The model under review builds one solid part; all positions refer to its coordinate system, in mm. Face numbers are marked on the shaded views. A direction names the side the tool comes from. Coordinates: 2 decimals unless noted, no trailing zeros. Order: outer loops, then holes, each group sorted by start corner. A loop starts at its lowest first (then second) coordinate and runs counter-clockwise, first axis right, second up. Notation, with made-up numbers: M 14,72 L 61,72 A14 cw 61,93 Z; hole C 41,-14.75 d4. An arc over 180 degrees is marked long. One line per item, written item: value.
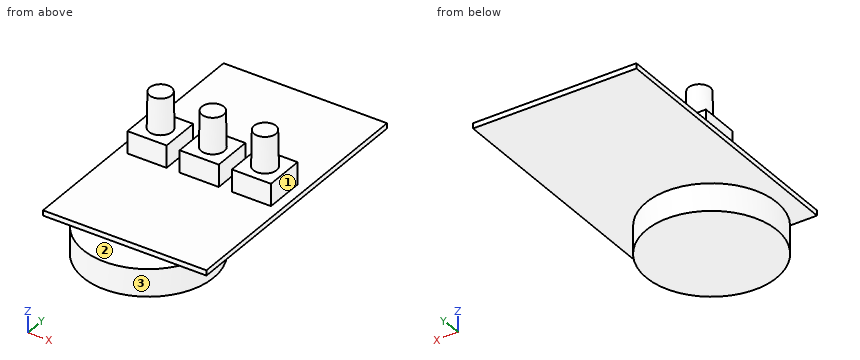
```python
from build123d import *

# Parameters (mm, degrees)
SKETCH_20_W                   = 25.05
SKETCH_20_H                   = 41.23
BOSS_EXTRUDE1_DEPTH           = 0.8
SKETCH13_W                    = 6
SKETCH13_H                    = 6.063806384
BOSS_EXTRUDE2_DEPTH           = 3.4
SKETCH14_R                    = 1.778
BOSS_EXTRUDE3_DEPTH           = 5.5
BOSS_EXTRUDE3_DRAFT           = 1
BOSS_EXTRUDE3_PROFILE_2_DEPTH = 5.5
BOSS_EXTRUDE3_PROFILE_2_DRAFT = 1
BOSS_EXTRUDE3_PROFILE_3_DEPTH = 5.5
BOSS_EXTRUDE3_PROFILE_3_DRAFT = 1
SKETCH15_R                    = 10
BOSS_EXTRUDE4_DEPTH           = 4.2


with BuildPart() as part:
    # Sketch 20 → Boss-Extrude1 (new body)
    with BuildSketch(Plane.XY):
        with Locations((12.525, 20.615)):
            Rectangle(SKETCH_20_W, SKETCH_20_H)
    extrude(amount=-BOSS_EXTRUDE1_DEPTH)

    # Sketch13 → Boss-Extrude2 (add)
    with BuildSketch(Plane.XY):
        with Locations((4.55409918, 20.007058513)):
            Rectangle(SKETCH13_W, SKETCH13_H)
        with Locations((12.546384712, 20.007058513)):
            Rectangle(SKETCH13_W, SKETCH13_H)
        with Locations((20.551668538, 20.007058513)):
            Rectangle(SKETCH13_W, SKETCH13_H)
    extrude(amount=BOSS_EXTRUDE2_DEPTH)


with BuildPart() as boss_extrude3_tool:
    # Sketch14 → Boss-Extrude3 (with draft: the straight prism first)
    with BuildSketch(Plane.XY.offset(3.4)):
        with Locations((4.6, 20)):
            Circle(SKETCH14_R)
    extrude(amount=BOSS_EXTRUDE3_DEPTH)
    # Boss-Extrude3: the draft: its side faces are tilted about the plane it starts from
    boss_extrude3_sides = [boss_extrude3_tool.faces().sort_by_distance(p)[0] for p in [
        (2.822, 20, 6.15),
    ]]
    draft(boss_extrude3_sides, Plane.XY.offset(3.4), BOSS_EXTRUDE3_DRAFT)


with BuildPart() as part_1:
    add(part.part)

    # Boss-Extrude3: add boss_extrude3_tool
    add(boss_extrude3_tool.part)


with BuildPart() as boss_extrude3_profile_2_tool:
    # Sketch14 → Boss-Extrude3 profile 2 (with draft: the straight prism first)
    with BuildSketch(Plane.XY.offset(3.4)):
        with Locations((12.6, 20)):
            Circle(SKETCH14_R)
    extrude(amount=BOSS_EXTRUDE3_PROFILE_2_DEPTH)
    # Boss-Extrude3 profile 2: the draft: its side faces are tilted about the plane it starts from
    boss_extrude3_profile_2_sides = [boss_extrude3_profile_2_tool.faces().sort_by_distance(p)[0] for p in [
        (10.822, 20, 6.15),
    ]]
    draft(boss_extrude3_profile_2_sides, Plane.XY.offset(3.4), BOSS_EXTRUDE3_PROFILE_2_DRAFT)


with BuildPart() as part_2:
    add(part_1.part)

    # Boss-Extrude3 profile 2: add boss_extrude3_profile_2_tool
    add(boss_extrude3_profile_2_tool.part)


with BuildPart() as boss_extrude3_profile_3_tool:
    # Sketch14 → Boss-Extrude3 profile 3 (with draft: the straight prism first)
    with BuildSketch(Plane.XY.offset(3.4)):
        with Locations((20.6, 20)):
            Circle(SKETCH14_R)
    extrude(amount=BOSS_EXTRUDE3_PROFILE_3_DEPTH)
    # Boss-Extrude3 profile 3: the draft: its side faces are tilted about the plane it starts from
    boss_extrude3_profile_3_sides = [boss_extrude3_profile_3_tool.faces().sort_by_distance(p)[0] for p in [
        (18.822, 20, 6.15),
    ]]
    draft(boss_extrude3_profile_3_sides, Plane.XY.offset(3.4), BOSS_EXTRUDE3_PROFILE_3_DRAFT)


with BuildPart() as part_3:
    add(part_2.part)

    # Boss-Extrude3 profile 3: add boss_extrude3_profile_3_tool
    add(boss_extrude3_profile_3_tool.part)

    # Sketch15 → Boss-Extrude4 (add)
    with BuildSketch(Plane.XY.offset(-0.8)):
        with Locations((12.51, 5.43)):
            Circle(SKETCH15_R)
    extrude(amount=-BOSS_EXTRUDE4_DEPTH)


solid = part_3.part
```
(1) For L1, parallel to Z at x = 21.75, y = 9.5; L2, parallel to Y at x = 4, z = 1.5; L3, parallel to Z at x = 6.5, y = 20, list the stretches that pass through material, from the lowest coordinate up.
Geometry results:
L1: z = -0.8 to 0
L2: y = 16.98 to 23.04
L3: z = -0.8 to 3.4
(2) We need section B-B, the plane z = 7.25. State the section outline as (x, y) points.
Geometry results:
outline: C 4.6,20 d3.42; C 12.6,20 d3.42; C 20.6,20 d3.42
(3) Insertion check: pin 1 Ø1 at (x, z) = (12, 2) entering from -Y; pin 2 Ø2.5 at (x, z) = (20, 2.5) entering from +Y; pin 3 Ø6 at (x, y) = (22.5, 8.5) entering from +Z; pin 4 Ø8 at (y, z) = (7, 7) entering from -X (3 decimals). Each pin has a flat end and moves straight along its axis. Give the tip position at first contact, or say it passes through.
Geometry results:
pin 1: stops at y = 16.98
pin 2: stops at y = 23.04
pin 3: stops at z = 0
pin 4: passes through
(4) Tool access review of the marked faces 1, 2 and 3: name each direction out of +Z, -Z, +X, -X, +Y, -Y from which nothing blocks a thin tool from reaching the whole face with its end or side.
Geometry results:
face 1: +Z, +X, +Y, -Y
face 2: +Z, +X, -X, -Y
face 3: -Z
(5) We need section C-C, the plane z = -3.75. State the section outline as (x, y) points.
Geometry results:
outline: C 12.51,5.43 d20
(6) We need section D-D, the plane y = 3.5. State the section outline as (x, z) points.
Geometry results:
outline: M 0,-0.8 L 2.7,-0.8 L 2.7,-5 L 22.32,-5 L 22.32,-0.8 L 25.05,-0.8 L 25.05,0 L 0,0 Z
(7) We need section A-A, the plane y = 26. State the section outline as (x, z) points.
Geometry results:
outline: M 0,-0.8 L 25.05,-0.8 L 25.05,0 L 0,0 Z
